For this review, take the finished solid that the model builds, in its own axes (mm). Give positions to 0.01 mm unless a question says otherwise; leave off trailing zeros. Loops run counter-clockwise (first coordinate to the right, second up) from the corner with the lowest first, then second, coordinate; pieces in that order, holes last. Notation, with made-up numbers: (18, -5) - (37, -5) arc R21 cw to (37, 30) - close; hole circle Ø1 at (-1.5, 55.25). An arc over 180 degrees is marked (long way). Use CSV: the item, a comma, the result in double quotes. Start each with the question number.
1. For pin 1 (1.5 mm diameter, centred on y = 1.5, z = 21.5, fed in from -X); pin 2 (1.5 mm diameter, centred on x = -16.5, y = 2, fed in from +Z), all flat-tipped, find the tip position at first contact; note any pin that passes through.
2. Wall thickness on line 1 (X direction, y = 2.25, z = 17); line 2 (X direction, y = 1.35, z = 7.5); line 3 (Z direction, x = -6.5, y = 1.4): over which ranges is each line inside the solid? List them lowest first.
3. Take a section at D-D on z = 20.5. Give the boundary of the cut face in (x, y), plus the area to 3 significant figures.
4. Take a section at A-A on x = -30. Give the boundary of the cut face in (y, z), plus the area to 3 significant figures.
5. Take a section at B-B on y = 1.5. State how many separate pieces and enclosed holes the cut face has, plus the area to 3 significant figures.
6. Take a section at C-C on z = 30. Give the boundary of the cut face in (x, y), plus the area to 3 significant figures.
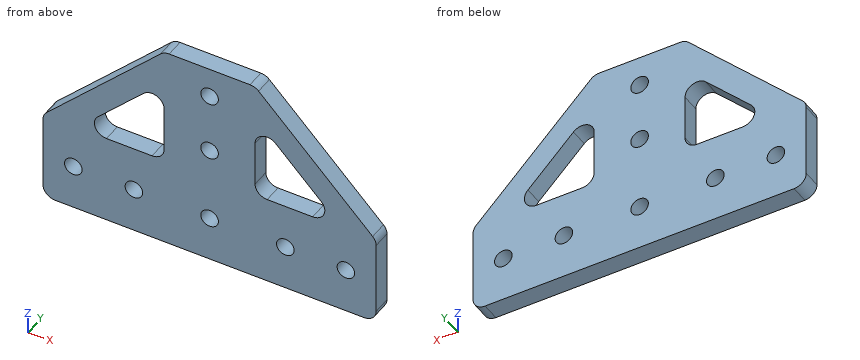
```python
from build123d import *

# Parameters (mm, degrees)
SKETCH_1_R      = 1.45
SKETCH_1_W      = 20
SKETCH_1_H      = 15
EXTRUDE_1_DEPTH = 3
EXTRUDE_2_DEPTH = 3
FILLET_1_R      = 2


with BuildPart() as part:
    # 草图1 → 凸台-拉伸1 (new body)
    # profile 1 of 2: a face of its own
    with BuildSketch(Plane(origin=(0, 0, 0), x_dir=(1, 0, 0), z_dir=(0, 1, 0))):
        Polygon((-15, -35), (-15, -15), (-35, -15), (-35, 0), (0, 0), (0, -35), align=None)
        with Locations(Location((-7.5, -30, 0), (0, 0, 270))):
            Circle(SKETCH_1_R, mode=Mode.SUBTRACT)
        with Locations(Location((-7.5, -20, 0), (0, 0, 270))):
            Circle(SKETCH_1_R, mode=Mode.SUBTRACT)
        with Locations(Location((-30, -7.5, 0), (0, 0, 270))):
            Circle(SKETCH_1_R, mode=Mode.SUBTRACT)
        with Locations(Location((-20, -7.5, 0), (0, 0, 270))):
            Circle(SKETCH_1_R, mode=Mode.SUBTRACT)
        with Locations(Location((-7.5, -7.5, 0), (0, 0, 270))):
            Circle(SKETCH_1_R, mode=Mode.SUBTRACT)
    # profile 2 of 2: a face of its own
    with BuildSketch(Plane(origin=(0, 0, 0), x_dir=(1, 0, 0), z_dir=(0, 1, 0))):
        with Locations((10, -7.5)):
            Rectangle(SKETCH_1_W, SKETCH_1_H)
        with Locations(Location((5, -7.5, 0), (0, 0, 270))):
            Circle(SKETCH_1_R, mode=Mode.SUBTRACT)
        with Locations(Location((15, -7.5, 0), (0, 0, 270))):
            Circle(SKETCH_1_R, mode=Mode.SUBTRACT)
    extrude(amount=EXTRUDE_1_DEPTH)

    # 草图2 → 凸台-拉伸2 (add)
    with BuildSketch(Plane(origin=(0, 3, 0), x_dir=(1, 0, 0), z_dir=(0, 1, 0))):
        Polygon((-35, -15), (-15, -35), (-15, -29.343145751), (-29.343145751, -15), align=None)
        Polygon((14.343145751, -15), (20, -15), (0, -35), (0, -29.343145751), align=None)
    extrude(amount=-EXTRUDE_2_DEPTH)

    # 圆角1
    fillet_1_edges = [part.edges().sort_by_distance(p)[0] for p in [
        (-15, 1.5, 15),
        (-35, 1.5, 15),
        (-35, 1.5, 0),
        (20, 1.5, 0),
        (20, 1.5, 15),
        (0, 1.5, 15),
        (0, 1.5, 35),
        (-15, 1.5, 35),
        (0, 1.5, 29.343145751),
        (14.343145751, 1.5, 15),
        (-29.343145751, 1.5, 15),
        (-15, 1.5, 29.343145751),
    ]]
    fillet(fillet_1_edges, radius=FILLET_1_R)


solid = part.part
```
Check result:
1,pin 1,"stops at x = -29.25"
1,pin 2,"stops at z = 34.25"
2,line 1,"x = -33 to -26.51, -15 to 0, 11.51 to 18"
2,line 2,"x = -35 to -31.45, -28.55 to -21.45, -18.55 to -8.95, -6.05 to 3.55, 6.45 to 13.55, 16.45 to 20"
2,line 3,"z = 0 to 6.45, 8.55 to 18.95, 21.05 to 28.95, 31.05 to 35"
3,outline,"(-29.5, 0) - (-23.84, 0) - (-23.84, 3) - (-29.5, 3) - close; (-15, 0) - (-8.86, 0) - (-8.86, 3) - (-15, 3) - close; (-6.14, 0) - (0, 0) - (0, 3) - (-6.14, 3) - close; (8.84, 0) - (14.5, 0) - (14.5, 3) - (8.84, 3) - close"
3,area,"70.8 mm²"
4,outline,"(0, 0) - (3, 0) - (3, 6.05) - (0, 6.05) - close; (0, 8.95) - (3, 8.95) - (3, 20) - (0, 20) - close"
4,area,"51.3 mm²"
5,separate pieces,"1"
5,enclosed holes,"9"
5,area,"1,290 mm²"
6,outline,"(-20, 0) - (-8.95, 0) - (-8.95, 3) - (-20, 3) - close; (-6.05, 0) - (5, 0) - (5, 3) - (-6.05, 3) - close"
6,area,"66.3 mm²"
